Check sheet for the modelled part. Datum: model origin and axes. Units: mm. A direction names the side the tool comes from. Round coordinates to 2 decimals unless told otherwise and drop trailing zeros. Use one line per item in the form item = value. Start each with the question number.
1) Gauge pin test, flat ends, axial feed: P1, Ø11.5, axis at x = 1.5, z = 34, coming from the -Y side; P2, Ø10.5, axis at y = 14.5, z = 35, coming from the -X side; P3, Ø12, axis at x = -26.5, y = 56.5, coming from the -Z side. Record the tip position at first contact, or that the pin passes through.
2) Section check A-A (z = 0). Count the separate pieces of the cut face and the enclosed holes in it, then the cut area to 3 significant figures.
3) Draft check along Z on faces 1 (the face through (-77.104, 88.07, -75.623)), 2 (the face through (76, 88, 0)), 3 (the face through (10, 10, 34)). Enter one of: +Z half, -Z half, draft (parallel to the pull), parting line (faces both ways), or undercut.
4) Scan lines: probe 1 along Z at (x, y) = (35.5, 20); probe 2 along Y at (x, z) = (20, -70); probe 3 along Z at (x, y) = (36, 20). Record each from-to range of solid material in increasing order.
5) Set-up check for faces 4 (the face through (97, 88, 10)), 5 (the face through (10, 88, 97)), 6 (the face through (0, 20, -35)): record each of +Z, -Z, +X, -X, +Y, -Y from which the full face is reachable in a straight line by a thin tool's end or side.
from build123d import *

# Parameters (mm, degrees)
SCHIZZO2_R                           = 10
TAGLIO_ESTRUSIONE2_DEPTH             = 10
RIPETIZIONECIRCOLARE2_COUNT          = 4
TAGLIO_ESTRUSIONE3_REACH             = 180.261
SCHIZZO4_R                           = 10
TAGLIO_ESTRUSIONE3_DIRECTION_2_REACH = 180.261
TAGLIO_ESTRUSIONE4_REACH             = 180.261
SCHIZZO5_W                           = 20
SCHIZZO5_H                           = 20
TAGLIO_ESTRUSIONE4_DIRECTION_2_REACH = 180.261


with BuildPart() as part:
    # Schizzo1 → Rivoluzione1 (revolve)
    with BuildSketch(Plane.XY, mode=Mode.PRIVATE) as rivoluzione1_sk:
        with BuildLine():
            Line((31, 0), (40, 0))
            Line((40, 0), (40, 45))
            ThreePointArc((40, 45), (55.192640723, 61.901498667), (63.638363359, 83))
            Line((63.638363359, 83), (108, 83))
            Line((108, 83), (108, 93))
            Line((108, 93), (55, 93))
            ThreePointArc((55, 93), (48.182091863, 67.998869263), (31, 48.6))
            Line((31, 48.6), (31, 0))
        make_face()
    revolve(rivoluzione1_sk.sketch.rotate(Axis((0, 136.24893985, 0), (0, -1, 0)), 180), axis=Axis((0, 136.24893985, 0), (0, -1, 0)))

    # Schizzo2 → Taglio-Estrusione2 (cut)
    with BuildSketch(Plane(origin=(0, 93, 0), x_dir=(1, 0, 0), z_dir=(0, 1, 0))):
        with Locations(Location((60.811183182, 60.811183182, 0), (0, 0, 180))):
            Circle(SCHIZZO2_R)
        with BuildLine():
            Line((107.53604047, 10), (86, 10))
            ThreePointArc((86, 10), (76, 0), (86, -10))
            Line((86, -10), (107.53604047, -10))
            ThreePointArc((107.53604047, -10), (108, 0), (107.53604047, 10))
        make_face()
    taglio_estrusione2 = extrude(amount=-TAGLIO_ESTRUSIONE2_DEPTH, mode=Mode.SUBTRACT)

    # RipetizioneCircolare2: Taglio-Estrusione2 ×4 about axis
    ripetizionecircolare2_axis = Axis((0, 0, 0), (0, 1, 0))
    for i in range(1, RIPETIZIONECIRCOLARE2_COUNT):
        add(taglio_estrusione2.rotate(ripetizionecircolare2_axis, i * 360 / RIPETIZIONECIRCOLARE2_COUNT), mode=Mode.SUBTRACT)

    # Schizzo4 → Taglio-Estrusione3 (cut, up to next)
    with BuildSketch(Plane(origin=(0, 0, 0), x_dir=(0, 0, -1), z_dir=(1, 0, 0)), mode=Mode.PRIVATE) as taglio_estrusione3_sk1:
        with Locations((0, 20)):
            Circle(SCHIZZO4_R)
    taglio_estrusione3_tool1 = extrude(taglio_estrusione3_sk1.sketch, amount=-TAGLIO_ESTRUSIONE3_REACH, mode=Mode.PRIVATE) & part.part
    add(taglio_estrusione3_tool1.solids().sort_by_distance((0, 20, 0))[0], mode=Mode.SUBTRACT)

    # Schizzo4 → Taglio-Estrusione3 direction 2 (cut, up to next)
    with BuildSketch(Plane(origin=(0, 0, 0), x_dir=(0, 0, -1), z_dir=(1, 0, 0)), mode=Mode.PRIVATE) as taglio_estrusione3_direction_2_sk1:
        with Locations((0, 20)):
            Circle(SCHIZZO4_R)
    taglio_estrusione3_direction_2_tool1 = extrude(taglio_estrusione3_direction_2_sk1.sketch, amount=TAGLIO_ESTRUSIONE3_DIRECTION_2_REACH, mode=Mode.PRIVATE) & part.part
    add(taglio_estrusione3_direction_2_tool1.solids().sort_by_distance((0, 20, 0))[0], mode=Mode.SUBTRACT)

    # Schizzo5 → Taglio-Estrusione4 (cut, up to next)
    with BuildSketch(Plane.XY, mode=Mode.PRIVATE) as taglio_estrusione4_sk1:
        with Locations((0, 10)):
            Rectangle(SCHIZZO5_W, SCHIZZO5_H)
    taglio_estrusione4_tool1 = extrude(taglio_estrusione4_sk1.sketch, amount=-TAGLIO_ESTRUSIONE4_REACH, mode=Mode.PRIVATE) & part.part
    add(taglio_estrusione4_tool1.solids().sort_by_distance((0, 10, 0))[0], mode=Mode.SUBTRACT)

    # Schizzo5 → Taglio-Estrusione4 direction 2 (cut, up to next)
    with BuildSketch(Plane.XY, mode=Mode.PRIVATE) as taglio_estrusione4_direction_2_sk1:
        with Locations((0, 10)):
            Rectangle(SCHIZZO5_W, SCHIZZO5_H)
    taglio_estrusione4_direction_2_tool1 = extrude(taglio_estrusione4_direction_2_sk1.sketch, amount=TAGLIO_ESTRUSIONE4_DIRECTION_2_REACH, mode=Mode.PRIVATE) & part.part
    add(taglio_estrusione4_direction_2_tool1.solids().sort_by_distance((0, 10, 0))[0], mode=Mode.SUBTRACT)


solid = part.part
Results are:
q1.P1 = 20
q1.P2 = -26.74
q1.P3 = -49.81
q2.separate_pieces = 4
q2.enclosed_holes = 0
q2.area = 1,700 mm²
q3.face_1 = -Z half
q3.face_2 = undercut
q3.face_3 = draft
q4.probe_1 = -18.43 to -10, 10 to 18.43
q4.probe_2 = 83 to 93
q4.probe_3 = -17.44 to -10, 10 to 17.44
q5.face_4 = +X, +Y, -Y
q5.face_5 = +Z, +Y, -Y
q5.face_6 = +Z, -Z, -Y
